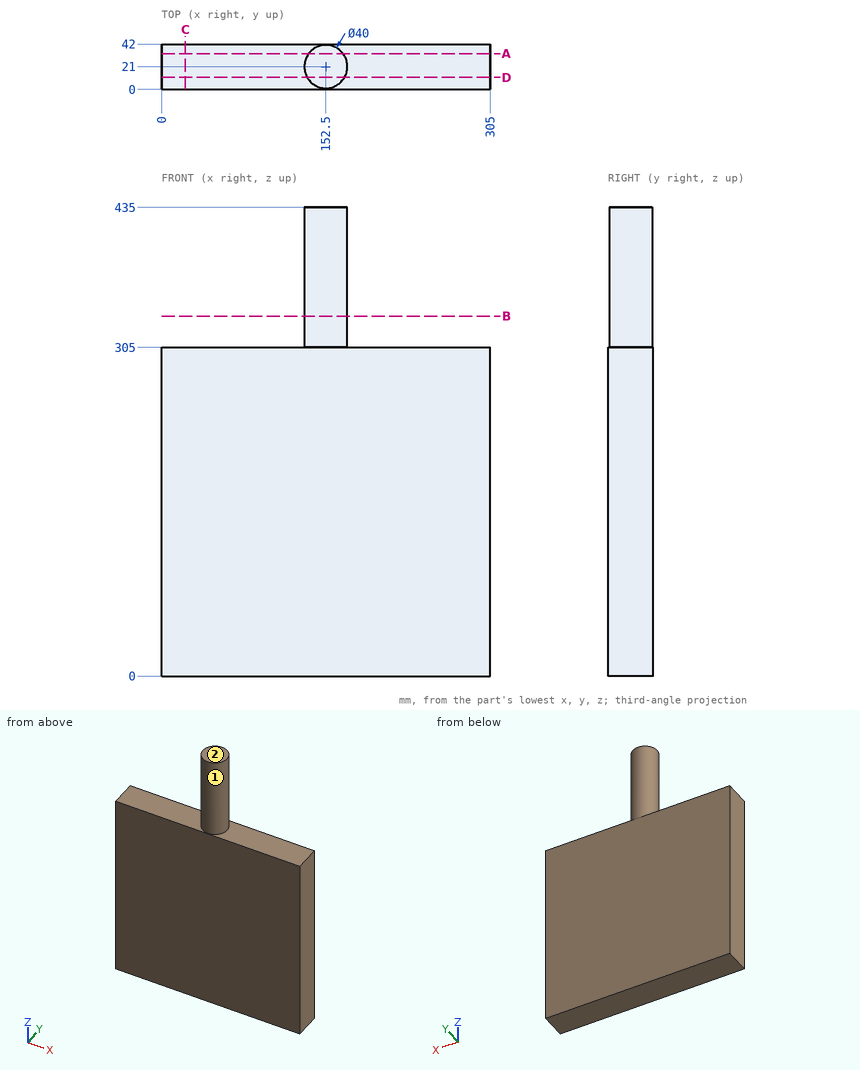
Study the drawing (mm; zero at the part's minimum x, y, z) and answer. A direction names the side the tool comes from. Give positions to 0.01 mm unless a question says otherwise; leave off trailing zeros. Order: outer loops, then holes, each group sorted by start corner. A loop starts at its lowest first (then second) coordinate and runs counter-clockwise, first axis right, second up. Notation, with made-up numbers: (-13.5, 81) - (18.5, 81) arc R25 cw to (18.5, 95) - close; hole circle Ø6 at (47.25, 81.5). An arc over 180 degrees is marked (long way). Answer in a Markdown table with one row per item. Add a question column.
Q1. Find the intervals of material crossed by line 1 along Z through (x, y) = (134, 30); line 2 along X through (y, z) = (28, 412) (3 decimals); line 3 along X through (y, z) = (15, 312.5), in increasing order. Write a range as [from, to].
Q2. Which of the six approach directions +Z, -Z, +X, -X, +Y, -Y give full straight-line access (tool end or side, diameter ignored) to the marked faces 1 and 2?
Q3. The part is cut by section D-D (y = 11). Determine the outline of the cut face in (x, z).
Q4. The part is cut by section A-A (y = 33). Determine the outline of the cut face in (x, z), then the cut area to 3 significant figures.
Q5. Given P1, Ø2, axis at y = 37, z = 143.5, coming from the -X side; P2, Ø1.5, axis at x = 256, y = 10.5, coming from the +Z side; P3, Ø1, axis at x = 171.5, z = 352, coming from the +Y side, each flat-ended and moving along its own axis, determine where each tip first touches the part or whether it passes through.
Q6. The part is cut by section C-C (x = 22). Determine the outline of the cut face in (y, z).
Q7. The part is cut by section B-B (z = 334). Determine the outline of the cut face in (x, y).
Determined:
| question | item | result |
|---|---|---|
| 1 | line 1 | z = [0, 305] |
| 1 | line 2 | x = [133.765, 171.235] |
| 1 | line 3 | x = [133.42, 171.58] |
| 2 | face 1 | +Z |
| 2 | face 2 | +Z, +X, -X, +Y, -Y |
| 3 | outline | (0, 0) - (305, 0) - (305, 305) - (169.82, 305) - (169.82, 435) - (135.18, 435) - (135.18, 305) - (0, 305) - close |
| 4 | outline | (0, 0) - (305, 0) - (305, 305) - (168.5, 305) - (168.5, 435) - (136.5, 435) - (136.5, 305) - (0, 305) - close |
| 4 | area | 97,200 mm² |
| 5 | P1 | stops at x = 0 |
| 5 | P2 | stops at z = 305 |
| 5 | P3 | stops at y = 28.6 |
| 6 | outline | (0, 0) - (42, 0) - (42, 305) - (0, 305) - close |
| 7 | outline | circle Ø40 at (152.5, 21) |
